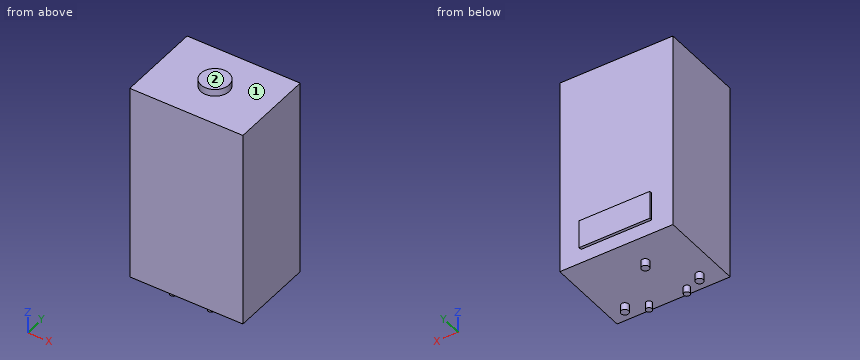
```python
from build123d import *

# Parameters (mm, degrees)
SKETCH_1_W      = 400
SKETCH_1_H      = 300
EXTRUDE_1_DEPTH = 702
SKETCH_2_R      = 13.4
SKETCH_2_R_2    = 10.65
EXTRUDE_2_DEPTH = 25
SKETCH_3_R      = 50
EXTRUDE_3_DEPTH = 25
SKETCH_4_W      = 250
SKETCH_4_H      = 100
EXTRUDE_4_DEPTH = 10


with BuildPart() as part:
    # Эскиз1 → Бобышка-Вытянуть1 (new body)
    with BuildSketch(Plane.XY):
        with Locations((200, 150)):
            Rectangle(SKETCH_1_W, SKETCH_1_H)
    extrude(amount=EXTRUDE_1_DEPTH)

    # Эскиз2 → Бобышка-Вытянуть2 (add)
    with BuildSketch(Plane(origin=(0, 0, 0), x_dir=(-1, 0, 0), z_dir=(0, 0, -1))):
        with Locations((-332, 60)):
            Circle(SKETCH_2_R)
        with Locations((-267, 30)):
            Circle(SKETCH_2_R_2)
        with Locations((-165, 200)):
            Circle(SKETCH_2_R)
        with Locations((-133, 30)):
            Circle(SKETCH_2_R_2)
        with Locations((-68, 60)):
            Circle(SKETCH_2_R)
    extrude(amount=EXTRUDE_2_DEPTH)

    # Эскиз3 → Бобышка-Вытянуть3 (add)
    with BuildSketch(Plane.XY.offset(702)):
        with Locations((200, 150)):
            Circle(SKETCH_3_R)
    extrude(amount=EXTRUDE_3_DEPTH)

    # Эскиз4 → Бобышка-Вытянуть4 (add)
    with BuildSketch(Plane(origin=(0, 300, 0), x_dir=(1, 0, 0), z_dir=(0, 1, 0))):
        with Locations((200, -100)):
            Rectangle(SKETCH_4_W, SKETCH_4_H)
    extrude(amount=EXTRUDE_4_DEPTH)


solid = part.part
```
Build history of the part. All positions in model axes, mm. Face numbers are marked on the shaded views. A direction names the side the tool comes from. Round coordinates to 2 decimals unless told otherwise and drop trailing zeros. Write each loop counter-clockwise with the first axis right and the second up, starting at its lowest first coordinate (ties: lowest second). Pieces come first, ordered by that corner, then holes.
1) Band-saw the part on A-A, the plane x = 267. List the corners of the cut face in (y, z), and give its area (3 significant figures).
2) Band-saw the part on C-C, the plane z = 493.5. List the corners of the cut face in (x, y).
3) Drill centre lines: probe 1 along Y at (x, z) = (360, 630); probe 2 along Z at (x, y) = (95.5, 267.5); probe 3 along Z at (x, y) = (236.5, 178.5). Where is each one in solid material? Low to high.
4) Band-saw the part on D-D, the plane y = 125.5. List the corners of the cut face in (x, z).
5) Pin check, flat tips, straight feed: pin 1 (12 mm diameter, centred on y = 105, z = 341.5, fed in from -X); pin 2 (1.5 mm diameter, centred on x = 153, y = 256, fed in from -Z); pin 3 (11 mm diameter, centred on y = 306, z = 92.5, fed in from -X); pin 4 (5 mm diameter, centred on x = 249.5, y = 303.5, fed in from -Z). Stop position of each tip, or through.
6) 3-axis set-ups, long thin cutter, end or side, ignore diameter. For the marked faces 1 and 2: which of +Z, -Z, +X, -X, +Y, -Y reach the whole face in a straight line?
7) Band-saw the part on B-B, the plane y = 30. List the corners of the cut face in (x, z), and give its area (3 significant figures).
Ans:
1. outline: (0, 0) - (19.35, 0) - (19.35, -25) - (40.65, -25) - (40.65, 0) - (300, 0) - (300, 50) - (310, 50) - (310, 150) - (300, 150) - (300, 702) - (0, 702) - close
1. area: 212,000 mm2
2. outline: (0, 0) - (400, 0) - (400, 300) - (0, 300) - close
3. probe 1: y = 0 to 300
3. probe 2: z = 0 to 702
3. probe 3: z = 0 to 727
4. outline: (0, 0) - (400, 0) - (400, 702) - (243.59, 702) - (243.59, 727) - (156.41, 727) - (156.41, 702) - (0, 702) - close
5. pin 1: stops at x = 0
5. pin 2: stops at z = 0
5. pin 3: stops at x = 75
5. pin 4: stops at z = 50
6. face 1: +Z
6. face 2: +Z, +X, -X, +Y, -Y
7. outline: (0, 0) - (122.35, 0) - (122.35, -25) - (143.65, -25) - (143.65, 0) - (256.35, 0) - (256.35, -25) - (277.65, -25) - (277.65, 0) - (400, 0) - (400, 702) - (0, 702) - close
7. area: 282,000 mm2
